The drawing under review shows one solid part. Ordinate dimensions are in mm from its lowest x, y, z. Round coordinates to 2 decimals unless told otherwise and drop trailing zeros. Write each loop counter-clockwise with the first axis right and the second up, starting at its lowest first coordinate (ties: lowest second). Pieces come first, ordered by that corner, then holes. Notation, with made-up numbers: (36, 19.5) -> (87, 19.5) arc R19 ccw to (87, 23.5) -> close; hole circle Ø3 at (87.5, 41.25). An arc over 180 degrees is marked (long way). Answer in a Markdown table with one row per item.
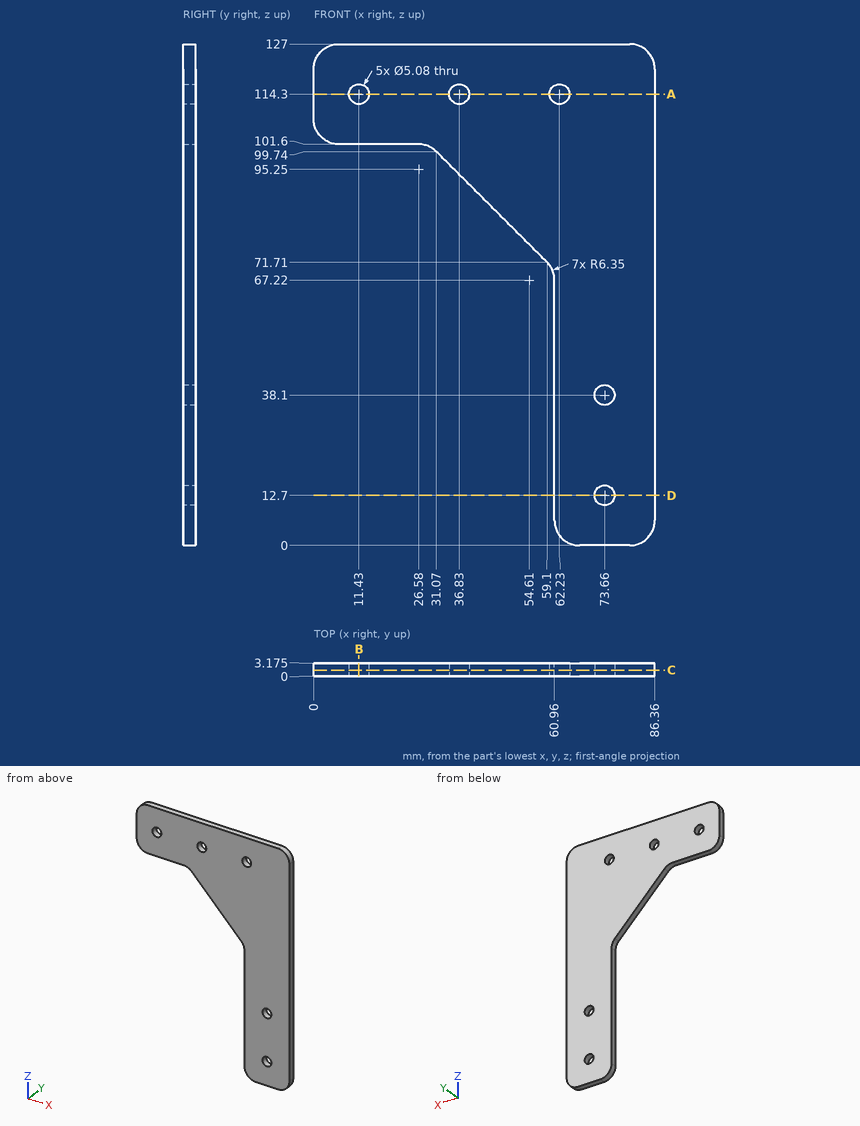
1) Consider section B-B on x = 11.43. State the section outline as (y, z) points (1 decimal).
Solved:
| item | result |
|---|---|
| outline | (0, 101.6) -> (3.2, 101.6) -> (3.2, 111.8) -> (0, 111.8) -> close; (0, 116.8) -> (3.2, 116.8) -> (3.2, 127) -> (0, 127) -> close |
2) Consider section A-A on z = 114.3. State the section outline as (x, y) points (1 decimal), then the cut area to 3 significant figures.
Solved:
| item | result |
|---|---|
| outline | (0, 0) -> (8.9, 0) -> (8.9, 3.2) -> (0, 3.2) -> close; (14, 0) -> (34.3, 0) -> (34.3, 3.2) -> (14, 3.2) -> close; (39.4, 0) -> (59.7, 0) -> (59.7, 3.2) -> (39.4, 3.2) -> close; (64.8, 0) -> (86.4, 0) -> (86.4, 3.2) -> (64.8, 3.2) -> close |
| area | 226 mm² |
3) For line 1 (X direction, y = 1.35, z = 114.3); line 2 (X direction, y = 1.55, z = 38.1); line 3 (X direction, y = 2.85, z = 48.5), list the stretches that pass through material, from the lowest coordinate up. Write a range as [from, to].
Solved:
| item | result |
|---|---|
| line 1 | [0, 8.89], [13.97, 34.29], [39.37, 59.69], [64.77, 86.36] |
| line 2 | [60.96, 71.12], [76.2, 86.36] |
| line 3 | [60.96, 86.36] |
4) Clearance check with a flat-ended pin moving along its axis: pin 1 Ø1.5 at (x, y) = (50, 2.5) entering from -Z. State where the tip first meets the part, or that it passes through.
Solved:
| item | result |
|---|---|
| pin 1 | z = 80.06 |
5) Consider section D-D on z = 12.7. State the section outline as (x, y) points (1 decimal), then the cut area to 3 significant figures.
Solved:
| item | result |
|---|---|
| outline | (61, 0) -> (71.1, 0) -> (71.1, 3.2) -> (61, 3.2) -> close; (76.2, 0) -> (86.4, 0) -> (86.4, 3.2) -> (76.2, 3.2) -> close |
| area | 64.5 mm² |
6) Consider section C-C on y = 1.5. State the section outline as (x, z) points.
Solved:
| item | result |
|---|---|
| outline | (0, 107.95) arc R6.35 ccw to (6.35, 101.6) -> (26.58, 101.6) arc R6.35 cw to (31.07, 99.74) -> (59.1, 71.71) arc R6.35 cw to (60.96, 67.22) -> (60.96, 6.35) arc R6.35 ccw to (67.31, 0) -> (80.01, 0) arc R6.35 ccw to (86.36, 6.35) -> (86.36, 120.65) arc R6.35 ccw to (80.01, 127) -> (6.35, 127) arc R6.35 ccw to (0, 120.65) -> close; hole circle Ø5.08 at (11.43, 114.3); hole circle Ø5.08 at (36.83, 114.3); hole circle Ø5.08 at (62.23, 114.3); hole circle Ø5.08 at (73.66, 12.7); hole circle Ø5.08 at (73.66, 38.1) |
